Can you work these out from the model? Positions are in its coordinate system, mm. A direction names the side the tool comes from. Round coordinates to 2 decimals unless told otherwise and drop trailing zeros. Write each loop counter-clockwise with the first axis right and the second up, starting at its lowest first coordinate (ties: lowest second). Pieces come first, ordered by that corner, then holes.
Q1. If we section it at C-C (y = -9.75): Please give me the cut outline in (x, z), plus the area to 3 significant figures.
Q2. I'm going to push flat-ended pins straight in: pin 1 Ø1.6 at (x, z) = (34, 4) entering from +Y; pin 2 Ø1.2 at (y, z) = (10.5, 4.5) entering from +X; pin 3 Ø1 at (y, z) = (-0.5, 4.5) entering from -X; pin 4 Ø1.9 at (x, y) = (7, 2.14) entering from +Z. Where does each tip first touch, or does it pass through?
Q3. If we section it at D-D (x = -3): Please give me the cut outline in (y, z).
Q4. Please list where these lines run through material, in increasing order: line 1 along Y through (x, z) = (7, 2.5); line 2 along Y through (x, z) = (30.5, 2.55); line 3 along Y through (x, z) = (20, 1.1).
Q5. We'd pull the mould along Z, two halves only. Please class faces 3 (the flat face through (15, 2, 0)), 4 (the cylindrical face through (36.52, -5.11, 1.52)), 5 (the flat face through (34, -3.571, 3)): +Z half, -Z half, draft (parallel to the pull), parting line (faces both ways), or undercut.
Q6. For faces 1 (the flat face through (34, 8.03, 3)), 2 (the flat face through (15, 2, 6)), which set-ups out of +Z, -Z, +X, -X, +Y, -Y let a thin tool reach every point of the face, with its end or its side?
Q7. If we section it at A-A (z = 0.85): Please give me the cut outline in (x, y).
Autodesk Inventor part; units mm, degrees
ref_plane "YZ Plane" through (0, 0, 0) normal (1, 0, 0) x (0, 1, 0)
ref_plane "XZ Plane" through (0, 0, 0) normal (0, 1, 0) x (-1, 0, 0)
ref_plane "XY Plane" through (0, 0, 0) normal (0, 0, 1) x (1, 0, 0)
ref_plane "작업 평면1" through (0, 0, 0) normal (0, 0, 1) x (1, 0, 0)
sketch "스케치1" plane through (0, 0, 0) normal (0, 0, 1) x (1, 0, 0)
  line L0 (6.993261, -11.657355) -> (26.993258, -11.667122)
  arc A0 (7.006739, 15.942642) -> (6.993261, -11.657355) centre (7, 2.142643) ccw
  line L1 (27.006737, 15.932875) -> (7.006739, 15.942642)
  line L2 (26.993258, -11.667122) -> (27.006737, 15.932875)
  circle A1 centre (-0.776779, -5.636927) radius 1.65
  circle A2 centre (-4, 2.140669) radius 1.65
  circle A3 centre (-0.77957, 9.919422) radius 1.65
  circle A4 centre (6.998026, 13.142643) radius 1.65
  circle A5 centre (14.776779, 9.922214) radius 1.65
  circle A6 centre (18, 2.144617) radius 1.65
  circle A7 centre (14.77957, -5.634135) radius 1.65
  circle A8 centre (7.001974, -8.857357) radius 1.65
  circle A9 centre (7, 2.142643) radius 5.1
  circle A10 centre (7, 2.142643) radius 3.55
  line L3 (6.99331, -11.557355) -> (26.993307, -11.567122)
  line L4 (26.993307, -11.567122) -> (27.006786, 16.032875)
  line L5 (27.006786, 16.032875) -> (7.006788, 16.042642)
  arc A11 (7.006788, 16.042642) -> (6.99331, -11.557355) centre (7.000049, 2.242643) ccw
  circle A12 centre (-0.781923, -5.531732) radius 1.65
  circle A13 centre (-3.99995, 2.248015) radius 1.65
  circle A14 centre (-0.774326, 10.024615) radius 1.65
  circle A15 centre (7.005421, 13.242642) radius 1.65
  circle A16 centre (14.782021, 10.017018) radius 1.65
  circle A17 centre (18.000048, 2.237271) radius 1.65
  circle A18 centre (14.774424, -5.539329) radius 1.65
  circle A19 centre (6.994677, -8.757356) radius 1.65
  circle A20 centre (7.000049, 2.242643) radius 5.1
  point P0 (0, 0)
  dimension "d0" = 7.1
extrude "돌출1" add sketch "스케치1" along normal blind 6 contours A11 L5 L4 L1 A0 | A0 L1 L2 L3 A11 | A1 A12 | A12 A1 | A1 A12 | A2 A13 | A13 A2 | A2 A13 | A14 A3 | A3 A14 | A3 A14 | A4 A15 | A4 A15 | A15 A4 | A5 A16 | A5 A16 | A16 A5 | A6 | A7 A18 | A18 A7 | A7 A18 | A8 A19 | A19 A8 | A8 A19 | A20 A9 | A9 A20 | A9 A20 | A17
offset faces "크기1" outward 2 faces at (10.504028, 1.573183, 4)
move faces "이동1" translate (4.999999, -0.002442, 0) faces at (27.00226, 6.766209, 4)
move faces "이동2" translate (1, -0.000488, 0) faces at (32.006753, 15.963766, 2) (32.00226, 6.763767, 4)
move faces "이동3" translate (4.999999, -0.002442, 0) faces at (33.006752, 15.963278, 2) (32.997783, -2.403387, 4)
sketch "스케치3" plane through (38.006784, 16.027503, 6) normal (0.9999999, -0.0004883, 0) x (0, 0, -1)
  circle A0 centre (3, -6) radius 1.55
  circle A1 centre (57.100995, -6.1) radius 1.55
  circle A2 centre (3, -21.6) radius 1.55
  circle A3 centre (57.100995, -21.7) radius 1.55
  line L0 (-17.781018, 8.082697) -> (114.718982, 8.082697)
  line L1 (-17.781018, -71.417303) -> (-17.781018, 8.082697)
  line L2 (114.718982, -71.417303) -> (-17.781018, -71.417303)
  line L3 (114.718982, 8.082697) -> (114.718982, -71.417303)
  point P0 (6, -16.046061)
extrude "돌출3" cut sketch "스케치3" against normal blind 10 contours A0 | A2
sketch "스케치4" plane through (0, 0, 0) normal (0, 0, -1) x (-1, 0, 0)
  line L0 (-38.006784, 16.027503) -> (-7.006788, 16.042642)
  line L1 (-33.358652, 16.029773) -> (-33.358652, 12.029773)
  line L2 (-33.358652, 16.029773) -> (-29.358652, 16.029773) construction
  line L3 (-6.99331, -11.557355) -> (-37.993306, -11.572494)
  line L4 (-34.023529, -11.570555) -> (-34.023529, -7.570555)
  line L5 (-34.023529, -11.570555) -> (-30.023529, -11.570555) construction
  line L6 (-37.993306, -11.572494) -> (-38.006784, 16.027503)
  line L7 (-37.995039, -8.023851) -> (-34.995039, -8.023851)
  line L8 (-37.995039, -8.023851) -> (-34.995039, -8.023851) construction
  line L9 (-34.995039, -7.570555) -> (-32.995039, -7.570555)
  line L10 (-32.995039, -7.570555) -> (-32.995039, -3.570555)
  line L11 (-32.995039, -3.570555) -> (-34.995039, -3.570555)
  line L12 (-34.995039, -3.570555) -> (-34.995039, -7.570555)
  line L13 (-34.995039, 12.029773) -> (-32.995039, 12.029773)
  line L14 (-32.995039, 12.029773) -> (-32.995039, 8.029773)
  line L15 (-32.995039, 8.029773) -> (-34.995039, 8.029773)
  line L16 (-34.995039, 8.029773) -> (-34.995039, 12.029773)
  point P0 (0, 0)
  dimension "d17" = 4
  dimension "d18" = 90
  dimension "d19" = 4
  dimension "d20" = 90
  dimension "d21" = 3
  dimension "d22" = 0
  dimension "d23" = 2
  dimension "d24" = 4
  dimension "d25" = 2
  dimension "d26" = 4
extrude "돌출4" cut sketch "스케치4" against normal blind 10
properties part number "6" material "아크릴, 선명"
A:
1. outline: (0.17, 0) - (37.99, 0) - (37.99, 6) - (0.17, 6) - close
1. area: 227 mm2
2. pin 1: stops at y = 16.03
2. pin 2: stops at x = 38
2. pin 3: stops at x = -6.62
2. pin 4: passes through
3. outline: (-7.27, 0) - (11.75, 0) - (11.75, 6) - (-7.27, 6) - close
4. line 1: y = -11.56 to 0.59, 3.69 to 16.04
4. line 2: y = -11.57 to -7.05, -4.09 to 8.55, 11.51 to 16.03
4. line 3: y = -11.56 to 16.04
5. face 3: -Z half
5. face 4: undercut
5. face 5: draft
6. face 1: +Z, -Z
6. face 2: +Z, +X, -X, +Y, -Y
7. outline: (6.99, -11.56) - (37.99, -11.57) - (38.01, 16.03) - (7.01, 16.04) arc R13.8 ccw to start; hole circle Ø3.1 at (7, 2.14); hole (33, -7.57) - (35, -7.57) - (35, -3.57) - (33, -3.57) - close; hole (33, 8.03) - (35, 8.03) - (35, 12.03) - (33, 12.03) - close
